Design review of the part built by this model. Coordinates are the model's own, in mm. Give positions to 0.01 mm unless a question says otherwise; leave off trailing zeros. Write each loop counter-clockwise with the first axis right and the second up, starting at its lowest first coordinate (ties: lowest second). Pieces come first, ordered by that corner, then holes. Notation, with made-up numbers: (66, -6) -> (125, -6) arc R9 ccw to (125, 7) -> close; hole circle Ø2 at (64.5, 74.25). An arc over 180 degrees is marked (long way). Put each result on its own line as item: value. Start each with the question number.
from build123d import *

# Parameters (mm, degrees)
F0_R     = 5
F1_DEPTH = 10


with BuildPart() as f1:
    # F0 (on Top) → F1 (new body)
    with BuildSketch(Plane.XY):
        with BuildLine():
            Line((159.43381, 15.66526), (-13.99655, 183.09931))
            ThreePointArc((-13.99655, 183.09931), (-38.831476, 185.45084), (-46.64062, 161.758636))
            Line((-46.64062, 161.758636), (-57.301475, 28.431364))
            Line((-57.301475, 28.431364), (0, -26.888927))
            Line((0, -26.888927), (147, -20))
            ThreePointArc((147, -20), (165.885248, -6.583875), (159.43381, 15.66526))
        make_face()
        Circle(F0_R, mode=Mode.SUBTRACT)
        with Locations((147, 0)):
            Circle(F0_R, mode=Mode.SUBTRACT)
        with Locations((-27.887755, 168.710619)):
            Circle(F0_R, mode=Mode.SUBTRACT)
    extrude(amount=F1_DEPTH)


solid = f1.part
Q1. Take a section at B-B on z = 7.25. Give the boundary of the cut face in (x, y), then the cut area to 3 significant figures.
Q2. Take a section at D-D on y = 76. Give the boundary of the cut face in (x, z), then the cut area to 3 significant figures.
Q3. To check wall thickness, follow probe 1 along X at (y, z) = (2.5, 3); probe 2 along Y at (x, z) = (147, 4.75); probe 3 along Y at (x, z) = (-24, 0.75). State the ranges of each line that lie inside material, in increasing order. Write a range as from..to.
Q4. Take a section at A-A on y = 0. Give the boundary of the cut face in (x, z).
Q5. Mouldability with a two-part tool opening along Y and no side actions: class faces 1 (the face through (-1.08, -4.88, 4.93)), 2 (the face through (73.933, 98.21, 4.93)), 3 (the face through (-29.052, 1.158, 4.93)) as +Y half, -Y half, draft (parallel to the pull), parting line (faces both ways), or undercut.
Q6. For pin 1 (1 mm diameter, centred on x = -29.5, z = 2.5, fed in from -Y); pin 2 (1 mm diameter, centred on x = 38, z = 6.5, fed in from -Y); pin 3 (6 mm diameter, centred on y = 23, z = 2.5, fed in from -X); pin 4 (9 mm diameter, centred on x = 0, y = 0, fed in from +Z), all flat-tipped, find the tip position at first contact; note any pin that passes through.
Q7. Take a section at C-C on x = 80. Give the boundary of the cut face in (y, z).
Result:
1. outline: (-57.3, 28.43) -> (0, -26.89) -> (147, -20) arc R20 ccw to (159.43, 15.67) -> (-14, 183.1) arc R20 ccw to (-46.64, 161.76) -> close; hole circle Ø10 at (-27.89, 168.71); hole circle Ø10 at (0, 0); hole circle Ø10 at (147, 0)
1. area: 27,900 mm^2
2. outline: (-53.5, 0) -> (96.94, 0) -> (96.94, 10) -> (-53.5, 10) -> close
2. area: 1,500 mm^2
3. probe 1: x = -30.44..-4.33, 4.33..142.67, 151.33..166.84
3. probe 2: y = -20..-5, 5..27.67
3. probe 3: y = -3.72..165.57, 171.85..188.33
4. outline: (-27.85, 0) -> (-5, 0) -> (-5, 10) -> (-27.85, 10) -> close; (5, 0) -> (142, 0) -> (142, 10) -> (5, 10) -> close; (152, 0) -> (167, 0) -> (167, 10) -> (152, 10) -> close
5. face 1: undercut
5. face 2: +Y half
5. face 3: -Y half
6. pin 1: stops at y = 1.11
6. pin 2: stops at y = -25.13
6. pin 3: stops at x = -54.78
6. pin 4: passes through
7. outline: (-23.14, 0) -> (92.35, 0) -> (92.35, 10) -> (-23.14, 10) -> close
